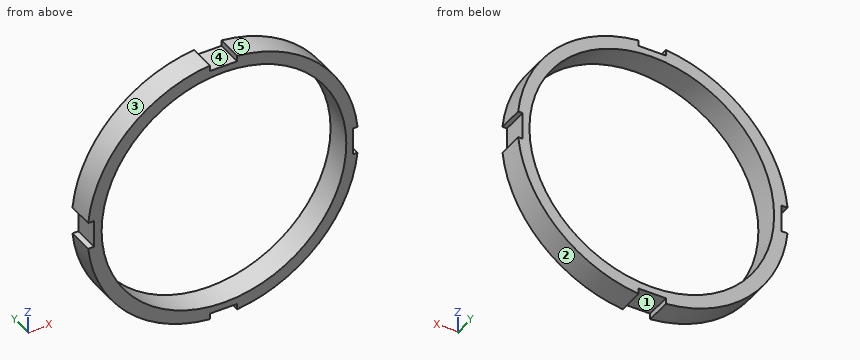
```python
from build123d import *

# Parameters (mm, degrees)
BOX004_W         = 10
BOX004_H         = 15
BOX004_DEPTH     = 10.5
BOX003_W         = 10
BOX003_H         = 15
BOX003_DEPTH     = 10.5
BOX002_W         = 10
BOX002_H         = 15
BOX002_DEPTH     = 10.5
BOX001_W         = 10
BOX001_H         = 15
BOX001_DEPTH     = 10.5
SKETCH017_R      = 52
SKETCH017_R_2    = 47
EXTRUDE004_DEPTH = 10


with BuildPart() as cube004:
    # Box004 → Box004 (new body)
    with BuildSketch(Plane(origin=(5.5, -12, 49.5), x_dir=(0, 0, 1), z_dir=(-1, 0, 0))):
        with Locations((5, 7.5)):
            Rectangle(BOX004_W, BOX004_H)
    extrude(amount=BOX004_DEPTH)


with BuildPart() as cube003:
    # Box003 → Box003 (new body)
    with BuildSketch(Plane(origin=(5.5, -12, -59.5), x_dir=(0, 0, 1), z_dir=(-1, 0, 0))):
        with Locations((5, 7.5)):
            Rectangle(BOX003_W, BOX003_H)
    extrude(amount=BOX003_DEPTH)


with BuildPart() as cube002:
    # Box002 → Box002 (new body)
    with BuildSketch(Plane(origin=(50, -12, -5.35), x_dir=(1, 0, 0), z_dir=(0, 0, 1))):
        with Locations((5, 7.5)):
            Rectangle(BOX002_W, BOX002_H)
    extrude(amount=BOX002_DEPTH)


with BuildPart() as cube001:
    # Box001 → Box001 (new body)
    with BuildSketch(Plane(origin=(-59.5, -12, -5.25), x_dir=(1, 0, 0), z_dir=(0, 0, 1))):
        with Locations((5, 7.5)):
            Rectangle(BOX001_W, BOX001_H)
    extrude(amount=BOX001_DEPTH)


with BuildPart() as brace_jig:
    # Sketch017 → Extrude004 (new body)
    with BuildSketch(Plane.XZ):
        Circle(SKETCH017_R)
        with Locations((0.427685, 0)):
            Circle(SKETCH017_R_2, mode=Mode.SUBTRACT)
    extrude(amount=EXTRUDE004_DEPTH)

    # Cut004: cut Cube001
    add(cube001.part, mode=Mode.SUBTRACT)

    # Cut005: cut Cube002
    add(cube002.part, mode=Mode.SUBTRACT)

    # Cut006: cut Cube003
    add(cube003.part, mode=Mode.SUBTRACT)

    # Cut007: cut Cube004
    add(cube004.part, mode=Mode.SUBTRACT)


solid = brace_jig.part
```
Read the model definition and answer for the solid it produces. Units are mm, in the model's axes. Face numbers are marked on the shaded views. A direction names the side the tool comes from. Round coordinates to 2 decimals unless told otherwise and drop trailing zeros. Loops run counter-clockwise (first coordinate to the right, second up) from the corner with the lowest first, then second, coordinate; pieces in that order, holes last. Notation, with made-up numbers: (21.5, 11.5) -> (64.5, 11.5) arc R12 cw to (64.5, 25.5) -> close; hole circle Ø3 at (-24, -14). An arc over 180 degrees is marked (long way). One line per item, written item: value.
1) A cutting plane is placed at B-B (y = -7.5). Determine the outline of the cut face in (x, z), and give its area (3 significant figures).
Answer list:
outline: (-51.73, -5.25) arc R52 ccw to (-5, -51.76) -> (-5, -49.5) -> (5.5, -49.5) -> (5.5, -51.71) arc R52 ccw to (51.72, -5.35) -> (50, -5.35) -> (50, 5.15) -> (51.74, 5.15) arc R52 ccw to (5.5, 51.71) -> (5.5, 49.5) -> (-5, 49.5) -> (-5, 51.76) arc R52 ccw to (-51.73, 5.25) -> (-49.5, 5.25) -> (-49.5, -5.25) -> close; hole circle Ø94 at (0.43, 0)
area: 1,460 mm²
2) Consider L1, parallel to X at y = -2.5, z = -33; L2, parallel to Z at x = -1.5, y = -5; L3, parallel to Z at x = 38, y = -1.75. Determine where each line is inside the solid, lowest interval first. Write a range as [from, to].
Answer list:
L1: x = [-40.19, -33.04], [33.89, 40.19]
L2: z = [-49.5, -46.96], [46.96, 49.5]
L3: z = [-35.5, -28.24], [28.24, 35.5]
3) The mould has two halves that part along X. Classify the marked faces 1, 2 and 3: pulls with the +X half, pulls with the -X half, needs draft (parallel to the pull), parting line crosses it, or undercut.
Answer list:
face 1: undercut
face 2: pulls with the +X half
face 3: pulls with the -X half
4) A cutting plane is placed at C-C (x = -28). Determine the outline of the cut face in (y, z).
Answer list:
outline: (-10, -43.82) -> (0, -43.82) -> (0, -37.43) -> (-10, -37.43) -> close; (-10, 37.43) -> (0, 37.43) -> (0, 43.82) -> (-10, 43.82) -> close
5) A cutting plane is placed at A-A (z = 0). Determine the outline of the cut face in (x, y), and give its area (3 significant figures).
Answer list:
outline: (-49.5, -10) -> (-46.57, -10) -> (-46.57, 0) -> (-49.5, 0) -> close; (47.43, -10) -> (50, -10) -> (50, 0) -> (47.43, 0) -> close
area: 55.0 mm²
6) For the marked faces 4 and 5, determine the directions among +Z, -Z, +X, -X, +Y, -Y from which every point of the face is accessible in a straight line to the end or side of a thin tool.
Answer list:
face 4: +Z, +Y, -Y
face 5: +Z, +X, +Y, -Y
7) Flat-ended cylindrical pins translate along their axes: P1, Ø1.5, axis at x = 34.5, z = -38, coming from the +Y side; P2, Ø5, axis at y = -7.5, z = -14.5, coming from the +X side; P3, Ø1.5, axis at y = -8, z = -32, coming from the -X side; P4, Ø6, axis at y = -2, z = 36.5, coming from the -X side. Find the tip coordinate at first contact, or state that the pin passes through.
Answer list:
P1: stops at y = 0
P2: stops at x = 50.6
P3: stops at x = -41.56
P4: stops at x = -39.77
